from build123d import *

# Parameters (mm, degrees)
F1_DEPTH = 2
F2_D     = 5
F2_DEPTH = 22.4
F2_TIP   = 1.5021515476
F3_D     = 4.2
F3_DEPTH = 22.4
F3_TIP   = 1.2618073
F4_D     = 5
F4_DEPTH = 22.4
F4_TIP   = 1.5021515476
F5_D     = 5
F5_DEPTH = 22.4
F5_TIP   = 1.5021515476


# Not quite as in the source:
# - a feature names something its author has since deleted; it is built from what else it names


with BuildPart() as f1:
    # F0 (on Top) → F1 (new body)
    with BuildSketch(Plane.XY):
        with BuildLine():
            Line((-19.0027786864, 90.978695631), (-154.5, 90.978695631))
            ThreePointArc((-154.5, 90.978695631), (-158.0355339059, 89.514229537), (-159.5, 85.978695631))
            Line((-159.5, 85.978695631), (-159.5, 55.978695631))
            Line((-159.5, 55.978695631), (-167.5, 55.978695631))
            ThreePointArc((-167.5, 55.978695631), (-171.0355339059, 54.514229537), (-172.5, 50.978695631))
            Line((-172.5, 50.978695631), (-172.5, -52.5))
            ThreePointArc((-172.5, -52.5), (-171.0355339059, -56.0355339059), (-167.5, -57.5))
            Line((-167.5, -57.5), (-159.5, -57.5))
            Line((-159.5, -57.5), (-159.5, -87.5))
            ThreePointArc((-159.5, -87.5), (-158.0355339059, -91.0355339059), (-154.5, -92.5))
            Line((-154.5, -92.5), (-19.364916731, -92.5))
            ThreePointArc((-19.364916731, -92.5), (-16.3030545526, -91.4528470752), (-14.5236875483, -88.75))
            ThreePointArc((-14.5236875483, -88.75), (0, -77.5), (14.5236875483, -88.75))
            ThreePointArc((14.5236875483, -88.75), (16.3030545526, -91.4528470752), (19.364916731, -92.5))
            Line((19.364916731, -92.5), (145.5, -92.5))
            ThreePointArc((145.5, -92.5), (149.0355339059, -91.0355339059), (150.5, -87.5))
            Line((150.5, -87.5), (150.5, 85.978695631))
            ThreePointArc((150.5, 85.978695631), (149.0355339059, 89.514229537), (145.5, 90.978695631))
            Line((145.5, 90.978695631), (19.0027786864, 90.978695631))
            ThreePointArc((19.0027786864, 90.978695631), (15.9500309398, 89.9385859319), (14.1673602092, 87.2509881092))
            ThreePointArc((14.1673602092, 87.2509881092), (0, 76.329125717), (-14.1673602092, 87.2509881092))
            ThreePointArc((-14.1673602092, 87.2509881092), (-15.9500309398, 89.9385859319), (-19.0027786864, 90.978695631))
        make_face()
    extrude(amount=F1_DEPTH)

    # F2
    with Locations(Plane(origin=(0, 0, 0), x_dir=(1, 0, 0), z_dir=(0, 0, -1))):
        with Locations((-104.5, -82.978695631), (95.5, -83.5), (162.5, -84.5), (140.5, 84.5), (95.5, 84.5), (-97.5, 84.5632106066), (-152.5, 84.5)):
            Hole(F2_D / 2, depth=F2_DEPTH)
            with Locations((0, 0, -(F2_DEPTH + F2_TIP / 2))):  # 118° drill point
                Cone(0, F2_D / 2, F2_TIP, mode=Mode.SUBTRACT)

    # F3
    with Locations(Plane(origin=(0, 0, 0), x_dir=(1, 0, 0), z_dir=(0, 0, -1))):
        with Locations((-97.5, 36.6775505245), (-152.5, 36.6775505245)):
            Hole(F3_D / 2, depth=F3_DEPTH)
            with Locations((0, 0, -(F3_DEPTH + F3_TIP / 2))):  # 118° drill point
                Cone(0, F3_D / 2, F3_TIP, mode=Mode.SUBTRACT)

    # F4
    with Locations(Plane(origin=(0, 0, 0), x_dir=(1, 0, 0), z_dir=(0, 0, -1))):
        with Locations((-164.5, -37.978695631), (-164.5, 39.5), (-104.5, 17.021304369), (0, 67.5), (0, -66.329125717), (95.5, -83.5), (95.5, 84.5), (140.5, 84.5), (162.5, -84.5)):
            Hole(F4_D / 2, depth=F4_DEPTH)
            with Locations((0, 0, -(F4_DEPTH + F4_TIP / 2))):  # 118° drill point
                Cone(0, F4_D / 2, F4_TIP, mode=Mode.SUBTRACT)

    # F5
    with Locations(Plane(origin=(0, 0, 0), x_dir=(1, 0, 0), z_dir=(0, 0, -1))):
        with Locations((-84.5, 84.5632106066)):
            Hole(F5_D / 2, depth=F5_DEPTH)
            with Locations((0, 0, -(F5_DEPTH + F5_TIP / 2))):  # 118° drill point
                Cone(0, F5_D / 2, F5_TIP, mode=Mode.SUBTRACT)


solid = f1.part
Read the model definition and answer for the solid it produces. Units are mm, in the model's axes. Coordinates: 2 decimals unless noted, no trailing zeros.
Q1. Consider probe 1 along Y at (x, z) = (-97.5, 1.5); probe 2 along Y at (x, z) = (-152.5, 1.6); probe 3 along Y at (x, z) = (-84.5, 1.1). Determine where each line is inside the solid, lowest interval first.
Q2. The mould has two halves that part along X. Classify faces 1 (the face through (-13, 1, 0)), 2 (the face through (0.27, 76.33, 0.99)): +X half, -X half, draft (parallel to the pull), parting line (faces both ways), or undercut.
Q3. The part is cut by section A-A on z = 0.6. Give the number of separate pieces and of enclosed holes in the cut face, and give its area (3 significant figures).
Q4. Each of these flat-tipped pins is pushed along its axis until it touches: pin 1 Ø4.5 at (x, y) = (0, 66.33) entering from +Z; pin 2 Ø1 at (y, z) = (-65.5, 1.5) entering from -X. Where does it stop, or does it pass through?
Results below:
1. probe 1: y = -92.5 to -87.06, -82.06 to -38.78, -34.58 to 90.98
1. probe 2: y = -92.5 to -87, -82 to -38.78, -34.58 to 90.98
1. probe 3: y = -92.5 to -87.06, -82.06 to 90.98
2. face 1: draft
2. face 2: undercut
3. separate pieces: 1
3. enclosed holes: 14
3. area: 57,400 mm2
4. pin 1: passes through
4. pin 2: stops at x = -159.5
